Part print with two shaded views. Sizes in mm from the minimum x, y, z corner. Coordinates: 2 decimals unless noted, no trailing zeros. Write each loop counter-clockwise with the first axis right and the second up, starting at its lowest first coordinate (ties: lowest second). Pieces come first, ordered by that corner, then holes. Notation, with made-up numbers: M -10,-29 L 0,-29 A13 cw 0,-11 Z; hole C -14,-23.5 d4. An arc over 180 degrees is marked long. One line per question, with ' | ' between items. Start each with the question number.
(1) Wall check: probe 1 along Z at (x, y) = (3, 14.25); probe 2 along Y at (x, z) = (7.5, 9.25). Give the ranges that are in metal, low to high.
(2) Cut at D-D (x = 3). Write the cut outline in (y, z).
(3) Cut at A-A (y = 8.5). Write the cut outline in (x, z), plus the area to 4 significant figures.
(4) Flat gauge pins, fed straight in: pin 1 Ø2 at (y, z) = (6.5, 12.5) entering from -X; pin 2 Ø3 at (y, z) = (3.5, 6.5) entering from +X; pin 3 Ø4 at (x, y) = (8.5, 8.5) entering from +Z; pin 4 Ø6 at (x, y) = (11, 11) entering from -Z. Where does each tip first touch, or does it go through?
(5) Cut at C-C (z = 14). Write the cut outline in (x, y).
(6) Two-plate mould, pull along Y, no slides. Class the marked faces 1, 2 and 3: +Y half, -Y half, draft (parallel to the pull), parting line (faces both ways), or undercut.
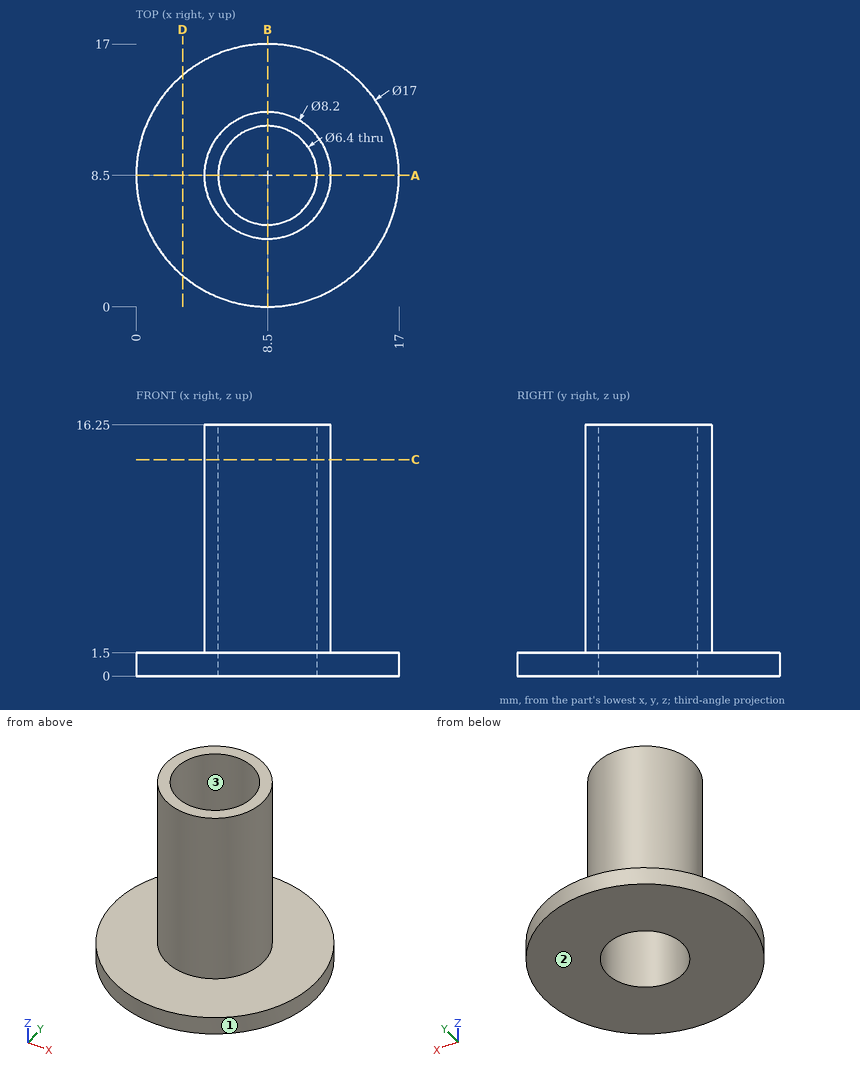
Filled in:
1) probe 1: 0 to 1.5 | probe 2: 4.52 to 5.46, 11.54 to 12.48
2) outline: M 2.02,0 L 14.98,0 L 14.98,1.5 L 2.02,1.5 Z
3) outline: M 0,0 L 5.3,0 L 5.3,16.25 L 4.4,16.25 L 4.4,1.5 L 0,1.5 Z; M 11.7,0 L 17,0 L 17,1.5 L 12.6,1.5 L 12.6,16.25 L 11.7,16.25 Z | area: 42.45 mm²
4) pin 1: x = 4.52 | pin 2: x = 10.64 | pin 3: through | pin 4: z = 0
5) outline: C 8.5,8.5 d8.2; hole C 8.5,8.5 d6.4
6) face 1: parting line | face 2: draft | face 3: undercut
